Build history of the part. All positions in model axes, mm. A direction names the side the tool comes from. Round coordinates to 2 decimals unless told otherwise and drop trailing zeros. Write each loop counter-clockwise with the first axis right and the second up, starting at its lowest first coordinate (ties: lowest second). Pieces come first, ordered by that corner, then holes. Notation, with made-up numbers: (8, 40.25) -> (48, 40.25) arc R14 ccw to (48, 57.25) -> close; hole circle Ø6 at (-27, 29.5). An arc over 180 degrees is marked (long way). Answer in a Markdown table with one row per item. Add a question column.
from build123d import *

# Parameters (mm, degrees)
BOSS_EXTRUDE1_DEPTH      = 15
BOSS_EXTRUDE1_DEPTH_BACK = 15
SKETCH1_W                = 45
SKETCH1_H                = 45
CUT_EXTRUDE1_DEPTH       = 12.75
CUT_EXTRUDE1_DEPTH_BACK  = 12.75
SKETCH2_W                = 38
SKETCH2_H                = 17
FILLET1_R                = 13
CUT_EXTRUDE2_REACH       = 54.5
SKETCH5_W                = 5
SKETCH5_H                = 16
FILLET2_R                = 2
CHAMFER3_SIZE            = 1.5
FILLET3_R                = 4


with BuildPart() as part:
    # Sketch1 → Boss-Extrude1 (new, two sides: drawn at the far end of the back side and taken through both)
    with BuildSketch(Plane(origin=(0, 0, 0), x_dir=(1, 0, 0), z_dir=(0, 1, 0)).offset(-BOSS_EXTRUDE1_DEPTH_BACK)):
        Rectangle(SKETCH1_W, SKETCH1_H)
    extrude(amount=BOSS_EXTRUDE1_DEPTH + BOSS_EXTRUDE1_DEPTH_BACK)

    # Sketch2 → Cut-Extrude1 (cut, two sides: drawn at the far end of the back side and taken through both)
    with BuildSketch(Plane(origin=(0, 0, 0), x_dir=(1, 0, 0), z_dir=(0, 1, 0)).offset(-CUT_EXTRUDE1_DEPTH_BACK)):
        with Locations((3.5, 11)):
            Rectangle(SKETCH2_W, SKETCH2_H)
        with Locations((3.5, -11)):
            Rectangle(SKETCH2_W, SKETCH2_H)
    extrude(amount=CUT_EXTRUDE1_DEPTH + CUT_EXTRUDE1_DEPTH_BACK, mode=Mode.SUBTRACT)

    # Fillet1
    # the kernel refuses this fillet: 13 mm, written as the material it adds along each edge
    with BuildSketch(Plane(origin=(-15.5, -12.75, -19.5), x_dir=(1, 0, 0), z_dir=(0, 0, 1))) as fillet1_piece_1_section:
        with BuildLine():
            CenterArc((FILLET1_R, FILLET1_R), FILLET1_R, 180, 90)
            Line((0, FILLET1_R), (0, 0))
            Line((0, 0), (FILLET1_R, 0))
        make_face()
    fillet1_piece_1 = extrude(amount=49.5, mode=Mode.PRIVATE)
    fillet1_piece_1 = split(fillet1_piece_1, bisect_by=Plane(origin=(-12.596216794, -9.846216794, 19.5), z_dir=(0, 0, -1)), keep=Keep.TOP, mode=Mode.PRIVATE)
    add(fillet1_piece_1)
    with BuildSketch(Plane(origin=(-15.5, 12.75, -19.5), x_dir=(1, 0, 0), z_dir=(0, 0, 1))) as fillet1_piece_2_section:
        with BuildLine():
            CenterArc((FILLET1_R, -FILLET1_R), FILLET1_R, 90, 90)
            Line((0, -FILLET1_R), (0, 0))
            Line((0, 0), (FILLET1_R, 0))
        make_face()
    fillet1_piece_2 = extrude(amount=49.5, mode=Mode.PRIVATE)
    fillet1_piece_2 = split(fillet1_piece_2, bisect_by=Plane(origin=(-12.596216794, 9.846216794, 19.5), z_dir=(0, 0, -1)), keep=Keep.TOP, mode=Mode.PRIVATE)
    add(fillet1_piece_2)
    with BuildSketch(Plane(origin=(-15.5, 12.75, 19.5), x_dir=(1, 0, 0), z_dir=(0, 0, -1))) as fillet1_piece_3_section:
        with BuildLine():
            CenterArc((FILLET1_R, FILLET1_R), FILLET1_R, 180, 90)
            Line((0, FILLET1_R), (0, 0))
            Line((0, 0), (FILLET1_R, 0))
        make_face()
    fillet1_piece_3 = extrude(amount=49.5, mode=Mode.PRIVATE)
    fillet1_piece_3 = split(fillet1_piece_3, bisect_by=Plane(origin=(-12.596216794, 9.846216794, -19.5), z_dir=(0, 0, 1)), keep=Keep.TOP, mode=Mode.PRIVATE)
    add(fillet1_piece_3)
    with BuildSketch(Plane(origin=(-15.5, -12.75, 19.5), x_dir=(1, 0, 0), z_dir=(0, 0, -1))) as fillet1_piece_4_section:
        with BuildLine():
            CenterArc((FILLET1_R, -FILLET1_R), FILLET1_R, 90, 90)
            Line((0, -FILLET1_R), (0, 0))
            Line((0, 0), (FILLET1_R, 0))
        make_face()
    fillet1_piece_4 = extrude(amount=49.5, mode=Mode.PRIVATE)
    fillet1_piece_4 = split(fillet1_piece_4, bisect_by=Plane(origin=(-12.596216794, -9.846216794, -19.5), z_dir=(0, 0, 1)), keep=Keep.TOP, mode=Mode.PRIVATE)
    add(fillet1_piece_4)

    # Sketch5 → Cut-Extrude2 (cut, up to next)
    with BuildSketch(Plane.XY.offset(22.5), mode=Mode.PRIVATE) as cut_extrude2_sk1:
        with Locations((20, 0)):
            Rectangle(SKETCH5_W, SKETCH5_H)
    cut_extrude2_tool1 = extrude(cut_extrude2_sk1.sketch, amount=-CUT_EXTRUDE2_REACH, mode=Mode.PRIVATE) & part.part
    cut_extrude2 = cut_extrude2_tool1.solids().sort_by_distance((20, 0, 22.5))[0]
    add(cut_extrude2, mode=Mode.SUBTRACT)

    # Mirror1: Cut-Extrude2 across plane
    add(cut_extrude2.mirror(Plane.XY), mode=Mode.SUBTRACT)

    # Fillet2
    fillet2_edges = [part.edges().sort_by_distance(p)[0] for p in [
        (0, 15, -22.5),
        (-22.5, 15, 0),
        (0, 15, 22.5),
        (0, -15, -22.5),
        (22.5, 15, 0),
        (-22.5, -15, 0),
        (0, -15, 22.5),
        (22.5, 11.5, 22.5),
        (-22.5, 0, 22.5),
        (-22.5, 0, -22.5),
        (22.5, -11.5, -22.5),
        (22.5, -11.5, 22.5),
        (22.5, 11.5, -22.5),
        (22.5, -15, 0),
    ]]
    fillet(fillet2_edges, radius=FILLET2_R)

    # Sketch3 → Revolve1 (revolve)
    with BuildSketch(Plane(origin=(0, 0, 0), x_dir=(1, 0, 0), z_dir=(0, 1, 0))):
        Polygon((-22.5, 0), (-32.5, 0), (-22.5, 5), align=None)
    revolve(axis=Axis((-22.5, 0, 0), (-1, 0, 0)))

    # Chamfer3
    # the kernel refuses this chamfer: 1.5 mm, written as the material it takes off along each edge
    with BuildSketch(Plane(origin=(22.5, 12.75, -19.5), x_dir=(0.0274958766105867, 0, -0.9996219169112968), z_dir=(0, -1, 0)), Plane(origin=(22.5, 4.142475518, 19.5), x_dir=(0.027495876610586768, 0, 0.9996219169112968), z_dir=(0, 1, 0))) as chamfer3_piece_1:
        Polygon((CHAMFER3_SIZE * 0.999621916911, -CHAMFER3_SIZE * 0.0274958766106), (-CHAMFER3_SIZE * 0.0274958766106, -CHAMFER3_SIZE * 0.999621916911), (0, 0), align=None)
    extrude(amount=8.607524482, mode=Mode.SUBTRACT)
    with BuildSketch(Plane(origin=(22.5, 12.75, -2.5), x_dir=(0.027495876610577594, 0, 0.999621916911297), z_dir=(0, -1, 0))) as chamfer3_piece_2:
        Polygon((CHAMFER3_SIZE * 0.999621916911, CHAMFER3_SIZE * 0.0274958766106), (-CHAMFER3_SIZE * 0.0274958766106, CHAMFER3_SIZE * 0.999621916911), (0, 0), align=None)
    extrude(amount=25.5, mode=Mode.SUBTRACT)
    with BuildSketch(Plane(origin=(22.5, 12.75, 2.5), x_dir=(0.027495876610577594, 0, -0.999621916911297), z_dir=(0, -1, 0))) as chamfer3_piece_3:
        Polygon((CHAMFER3_SIZE * 0.999621916911, -CHAMFER3_SIZE * 0.0274958766106), (-CHAMFER3_SIZE * 0.0274958766106, -CHAMFER3_SIZE * 0.999621916911), (0, 0), align=None)
    extrude(amount=25.5, mode=Mode.SUBTRACT)

    # Fillet3
    fillet3_edges = [part.edges().sort_by_distance(p)[0] for p in [
        (17.5, -8, -21),
        (17.5, 8, -21),
        (17.5, -8, 21),
        (17.5, 8, 21),
    ]]
    fillet(fillet3_edges, radius=FILLET3_R)


solid = part.part
(1) Saw through at C-C (y = 10). List the corners of the cut face in (x, z).
(2) Which spindle directions (+Z, -Z, +X, -X, +Y, -Y) get a long thin tool onto all of the face, cutting with end or side? Do faces 4 (the face through (17.5, 0, -21)), 5 (the face through (10, 12.75, 11)), 6 (the face through (0, 0, 22.5)), 7 (the face through (18.641, -6.797, 20.979)), 8 (the face through (21.93, 10.47, -21.9)). Say none if no direction does.
(3) Saw through at A-A (x = 4.5). List the corners of the cut face in (y, z), plus the area to 3 significant figures.
(4) Drop flat-ended pins along their axis: P1, Ø2, axis at y = -8, z = -15.5, coming from the +X side; P2, Ø0.8, axis at x = 22, z = -21, coming from the +Y side; P3, Ø8, axis at x = -25, y = -5, coming from the +Z side. Give the stop position or say it passes through.
(5) Probe line 1 along Z through (x, y) = (6, 10.75); line 2 along Y through (x, z) = (10, -11); line 3 along Y through (x, z) = (-5, -6.5). List the from-to ranges inside material, lowest first.
(6) Saw through at B-B (z = 13). List the corners of the cut face in (x, y).
(7) Saw through at D-D (x = -12). List the corners of the cut face in (y, z).
(8) Mould opens along Y. For faces 1 (the face through (-28.54, -0.59, -1.89)), 2 (the face through (21.93, -10.4, -21.9)), 3 (the face through (18.703, 6.859, 20.979)) say: pulls with the +Y half, pulls with the -Y half, needs draft (parallel to the pull), parting line crosses it, or undercut.
Answer sheet:
| question | item | result |
|---|---|---|
| 1 | outline | (-22.5, -20.5) arc R2 ccw to (-20.5, -22.5) -> (20.5, -22.5) arc R2 ccw to (22.45, -20.95) -> (21, -19.5) -> (-10.5, -19.5) -> (-10.5, -2.5) -> (21, -2.5) -> (22.5, -1) -> (22.5, 1) -> (21, 2.5) -> (-10.5, 2.5) -> (-10.5, 19.5) -> (21, 19.5) -> (22.45, 20.95) arc R2 ccw to (20.5, 22.5) -> (-20.5, 22.5) arc R2 ccw to (-22.5, 20.5) -> close |
| 2 | face 4 | -Z, +X |
| 2 | face 5 | +X |
| 2 | face 6 | +Z, +X, -X, +Y, -Y |
| 2 | face 7 | +Z, +X |
| 2 | face 8 | -Z, +X, +Y, -Y |
| 3 | outline | (-15, -20.5) arc R2 ccw to (-13, -22.5) -> (13, -22.5) arc R2 ccw to (15, -20.5) -> (15, 20.5) arc R2 ccw to (13, 22.5) -> (-13, 22.5) arc R2 ccw to (-15, 20.5) -> close; hole (-12.75, -19.5) -> (12.75, -19.5) -> (12.75, -2.5) -> (-12.75, -2.5) -> close; hole (-12.75, 2.5) -> (12.75, 2.5) -> (12.75, 19.5) -> (-12.75, 19.5) -> close |
| 3 | area | 480 mm² |
| 4 | P1 | stops at x = -11.63 |
| 4 | P2 | stops at y = 14.61 |
| 4 | P3 | stops at z = 22.44 |
| 5 | line 1 | z = -22.5 to -19.5, -2.5 to 2.5, 19.5 to 22.5 |
| 5 | line 2 | y = -15 to -12.75, 12.75 to 15 |
| 5 | line 3 | y = -15 to -12.51, 12.51 to 15 |
| 6 | outline | (-22.5, -13) arc R2 ccw to (-20.5, -15) -> (20.5, -15) arc R2 ccw to (22.5, -13) -> (22.5, -12.75) -> (-2.5, -12.75) arc R13 cw to (-15.5, 0) arc R13 cw to (-2.5, 12.75) -> (22.5, 12.75) -> (22.5, 13) arc R2 ccw to (20.5, 15) -> (-20.5, 15) arc R2 ccw to (-22.5, 13) -> close |
| 7 | outline | (-15, -20.5) arc R2 ccw to (-13, -22.5) -> (13, -22.5) arc R2 ccw to (15, -20.5) -> (15, 20.5) arc R2 ccw to (13, 22.5) -> (-13, 22.5) arc R2 ccw to (-15, 20.5) -> close; hole (-8.62, -19.5) -> (8.62, -19.5) -> (8.62, -2.5) -> (-8.62, -2.5) -> close; hole (-8.62, 2.5) -> (8.62, 2.5) -> (8.62, 19.5) -> (-8.62, 19.5) -> close |
| 8 | face 1 | parting line crosses it |
| 8 | face 2 | needs draft |
| 8 | face 3 | undercut |
